from build123d import *

# Parameters (mm, degrees)
BOSS_EXTRUDE1_DEPTH = 90
CUT_EXTRUDE1_DEPTH  = 51.8
SKETCH3_R           = 2.1
SKETCH3_R_2         = 3
CUT_EXTRUDE2_DEPTH  = 51.8
SKETCH4_R           = 2.5
CUT_EXTRUDE3_DEPTH  = 100.821221194


with BuildPart() as part:
    # Sketch1 → Boss-Extrude1 (new body)
    with BuildSketch(Plane(origin=(0, 0, 0), x_dir=(0, 0, -1), z_dir=(1, 0, 0))):
        Polygon((0, 0), (0, 100), (1.5875, 100), (1.5875, 1.5875), (50.8, 1.5875), (50.8, 0), align=None)
    extrude(amount=BOSS_EXTRUDE1_DEPTH)

    # Sketch2 → Cut-Extrude1 (cut, through all)
    with BuildSketch(Plane.XY):
        with BuildLine():
            Line((35.064378218, 94.92), (0, 49.2))
            Line((0, 49.2), (0, 100))
            Line((0, 100), (90, 100))
            Line((90, 100), (90, 49.2))
            Line((90, 49.2), (54.935621782, 94.92))
            ThreePointArc((54.935621782, 94.92), (45, 99.821221194), (35.064378218, 94.92))
        make_face()
    extrude(amount=-CUT_EXTRUDE1_DEPTH, mode=Mode.SUBTRACT)

    # Sketch3 → Cut-Extrude2 (cut, through all)
    with BuildSketch(Plane.XY):
        with Locations((45, 87.121221194)):
            Circle(SKETCH3_R)
        with Locations((65.784609691, 51.121221194)):
            Circle(SKETCH3_R)
        with Locations((24.215390309, 51.121221194)):
            Circle(SKETCH3_R)
        with Locations((45, 63.121221194)):
            Circle(SKETCH3_R_2)
    extrude(amount=-CUT_EXTRUDE2_DEPTH, mode=Mode.SUBTRACT)

    # Sketch4 → Cut-Extrude3 (cut, through all)
    with BuildSketch(Plane.XZ):
        with Locations((15, -16.3875)):
            Circle(SKETCH4_R)
        with Locations((75, -16.3875)):
            Circle(SKETCH4_R)
    extrude(amount=-CUT_EXTRUDE3_DEPTH, mode=Mode.SUBTRACT)


solid = part.part
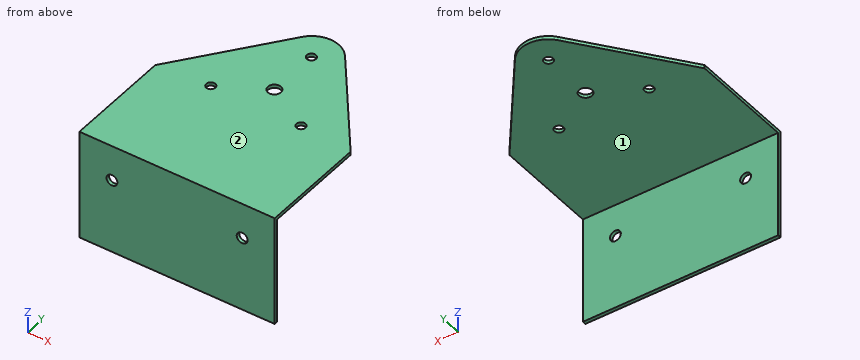
Can you work these out from the model? Positions are in its coordinate system, mm. Face numbers are marked on the shaded views. A direction names the side the tool comes from. Round coordinates to 2 decimals unless told otherwise and drop trailing zeros. Loops run counter-clockwise (first coordinate to the right, second up) from the corner with the lowest first, then second, coordinate; pieces in that order, holes last. Notation, with made-up numbers: (53, 64.5) - (94, 64.5) arc R14 cw to (94, 80.5) - close; hole circle Ø6 at (13, 40.25). An arc over 180 degrees is marked (long way). Use CSV: the item, a comma, the result in double quotes. Start each with the question number.
1) For the marked faces 1 and 2, which set-ups out of +Z, -Z, +X, -X, +Y, -Y let a thin tool reach every point of the face, with its end or its side?
2) If we section it at D-D on z = -44: Write out the boundary of the cut face in (x, y).
3) For pin 1 Ø6.5 at (x, y) = (45, 87.12) entering from -Z; pin 2 Ø3 at (x, z) = (75, -16.39) entering from +Y; pin 3 Ø3 at (x, z) = (22, -42.5) entering from +Y, each with a flat end and sliding along its axis, tell me the tip position at first contact or that it passes through.
4) If we section it at B-B on x = 75: Write out the boundary of the cut face in (y, z).
5) Please list where these lines run through material, in increasing order: probe 1 along Y at (x, z) = (45, -1.2); probe 2 along Z at (x, y) = (15, 1); probe 3 along Z at (x, y) = (15.5, 31.5). Write a range as [from, to].
6) If we section it at C-C on y = 15: Write out the boundary of the cut face in (x, z).
7) If we section it at A-A on x = 45: Write out the boundary of the cut face in (y, z), plus the area to 3 significant figures.
Geometry results:
1,face 1,"-Z, +X, -X, +Y"
1,face 2,"+Z, +X, -X, +Y, -Y"
2,outline,"(0, 0) - (90, 0) - (90, 1.59) - (0, 1.59) - close"
3,pin 1,"stops at z = -1.59"
3,pin 2,"passes through"
3,pin 3,"stops at y = 1.59"
4,outline,"(0, -50.8) - (1.59, -50.8) - (1.59, -18.89) - (0, -18.89) - close; (0, -13.89) - (1.59, -13.89) - (1.59, -1.59) - (68.76, -1.59) - (68.76, 0) - (0, 0) - close"
5,probe 1,"y = [0, 60.12], [66.12, 85.02], [89.22, 99.82]"
5,probe 2,"z = [-50.8, -18.89], [-13.89, 0]"
5,probe 3,"z = [-1.59, 0]"
6,outline,"(0, -1.59) - (90, -1.59) - (90, 0) - (0, 0) - close"
7,outline,"(0, -50.8) - (1.59, -50.8) - (1.59, -1.59) - (60.12, -1.59) - (60.12, 0) - (0, 0) - close; (66.12, -1.59) - (85.02, -1.59) - (85.02, 0) - (66.12, 0) - close; (89.22, -1.59) - (99.82, -1.59) - (99.82, 0) - (89.22, 0) - close"
7,area,"220 mm2"
